```python
from build123d import *

# Parameters (mm, degrees)
CROQUIS1_R              = 2.2
SALIENTE_EXTRUIR1_DEPTH = 8.3
CORTAR_EXTRUIR1_DEPTH   = 10
CROQUIS3_R              = 11.19
CROQUIS3_R_2            = 2.2
SALIENTE_EXTRUIR2_DEPTH = 3
REDONDEO1_R             = 10
REDONDEO2_R             = 10


with BuildPart() as part:
    # Croquis1 → Saliente-Extruir1 (new body)
    with BuildSketch(Plane.XY):
        with BuildLine():
            ThreePointArc((-1.855132773, 21.210566025), (0.747663665, 19.413438157), (3.480969897, 21.005058374))
            ThreePointArc((3.480969897, 21.005058374), (4.187425829, 21.678765959), (5.158862158, 21.775064198))
            ThreePointArc((5.158862158, 21.775064198), (8.457254598, 20.718159287), (11.553044037, 19.164927682))
            ThreePointArc((11.553044037, 19.164927682), (12.17958806, 18.416325998), (12.212774884, 17.4406926))
            ThreePointArc((12.212774884, 17.4406926), (13.051461105, 14.390967482), (16.16836891, 13.853283925))
            ThreePointArc((16.16836891, 13.853283925), (17.142596439, 13.915272757), (17.948659156, 13.364614252))
            ThreePointArc((17.948659156, 13.364614252), (19.796008974, 10.434812326), (21.16912324, 7.255032793))
            ThreePointArc((21.16912324, 7.255032793), (21.16789192, 6.278835898), (20.566189442, 5.510125275))
            ThreePointArc((20.566189442, 5.510125275), (19.248334843, 2.634803184), (21.290408418, 0.219403966))
            ThreePointArc((21.290408418, 0.219403966), (22.076555656, -0.359331218), (22.340079057, -1.299287234))
            ThreePointArc((22.340079057, -1.299287234), (21.871990743, -4.731099292), (20.879934411, -8.049572571))
            ThreePointArc((20.879934411, -8.049572571), (20.251503896, -8.796591301), (19.296455393, -8.998690904))
            ThreePointArc((19.296455393, -8.998690904), (16.438698786, -10.354214806), (16.450429211, -13.517137548))
            ThreePointArc((16.450429211, -13.517137548), (16.680649129, -14.465800124), (16.278327685, -15.355237783))
            ThreePointArc((16.278327685, -15.355237783), (13.713824964, -17.683276971), (10.820792216, -19.587693468))
            ThreePointArc((10.820792216, -19.587693468), (9.859212129, -19.755995666), (8.997695409, -19.2969196))
            ThreePointArc((8.997695409, -19.2969196), (5.937212872, -18.498380614), (3.91311135, -20.928860176))
            ThreePointArc((3.91311135, -20.928860176), (3.479681489, -21.803560382), (2.599765876, -22.226301918))
            ThreePointArc((2.599765876, -22.226301918), (-0.861191929, -22.361252828), (-4.301518916, -21.960514898))
            ThreePointArc((-4.301518916, -21.960514898), (-5.146314566, -21.471350096), (-5.511186255, -20.565905154))
            ThreePointArc((-5.511186255, -20.565905154), (-7.34236093, -17.986948546), (-10.455194801, -18.54773653))
            ThreePointArc((-10.455194801, -18.54773653), (-11.349467792, -18.939192417), (-12.29525528, -18.697432369))
            ThreePointArc((-12.29525528, -18.697432369), (-15.033247546, -16.576149969), (-17.411101542, -14.057767343))
            ThreePointArc((-17.411101542, -14.057767343), (-17.743823481, -13.140021189), (-17.44132262, -12.211875121))
            ThreePointArc((-17.44132262, -12.211875121), (-17.186362452, -9.059223351), (-19.931399108, -7.487920827))
            ThreePointArc((-19.931399108, -7.487920827), (-20.868074958, -7.212965835), (-21.437189843, -6.419826415))
            ThreePointArc((-21.437189843, -6.419826415), (-22.171079561, -3.034882316), (-22.373836253, 0.422765786))
            ThreePointArc((-22.373836253, 0.422765786), (-22.038800189, 1.339669668), (-21.210470293, 1.856227))
            ThreePointArc((-21.210470293, 1.856227), (-18.988673977, 4.107413132), (-20.08148026, 7.075576251))
            ThreePointArc((-20.08148026, 7.075576251), (-20.622277928, 7.888287624), (-20.548425031, 8.861687667))
            ThreePointArc((-20.548425031, 8.861687667), (-18.934817045, 11.926440502), (-16.867604324, 14.705482106))
            ThreePointArc((-16.867604324, 14.705482106), (-16.021577354, 15.192514199), (-15.055003187, 15.055779879))
            ThreePointArc((-15.055003187, 15.055779879), (-11.905973913, 15.352145362), (-10.835213617, 18.328332564))
            ThreePointArc((-10.835213617, 18.328332564), (-10.727087865, 19.298523636), (-10.044823777, 19.996719603))
            ThreePointArc((-10.044823777, 19.996719603), (-6.838743197, 21.307249261), (-3.468832869, 22.107339915))
            ThreePointArc((-3.468832869, 22.107339915), (-2.507680415, 21.936612489), (-1.855132773, 21.210566025))
        make_face()
        with Locations(Location((0, 0, 0), (0, 0, 180))):
            Circle(CROQUIS1_R, mode=Mode.SUBTRACT)
    extrude(amount=SALIENTE_EXTRUIR1_DEPTH)

    # Croquis2 → Cortar-Extruir1 (cut)
    with BuildSketch(Plane.XY.offset(8.3)):
        Polygon((7.216878365, 0), (3.608439182, 6.25), (-3.608439182, 6.25), (-7.216878365, 0), (-3.608439182, -6.25), (3.608439182, -6.25), align=None)
    extrude(amount=-CORTAR_EXTRUIR1_DEPTH, mode=Mode.SUBTRACT)

    # Croquis3 → Saliente-Extruir2 (add)
    with BuildSketch(Plane(origin=(0, 0, 0), x_dir=(-1, 0, 0), z_dir=(0, 0, -1))):
        with Locations(Location((0, 0, 0), (0, 0, 180))):
            Circle(CROQUIS3_R)
        Circle(CROQUIS3_R_2, mode=Mode.SUBTRACT)
    extrude(amount=SALIENTE_EXTRUIR2_DEPTH)

    # Redondeo1
    # the kernel refuses this fillet: 10 mm, written as the material it adds along each edge
    with BuildSketch(Plane(origin=(0, 0, 0), x_dir=(1, 0, 0), z_dir=(0, 1, 0))) as redondeo1_piece_1:
        with BuildLine():
            CenterArc((18.331428429, 10), REDONDEO1_R, 224.427004001, 45.572995999)
            Line((11.19, 3), (11.047171431, 2.86))
            ThreePointArc((11.047171431, 2.86), (10.99, 1.5), (10.99, 0))
            Line((10.99, 0), (11.19, -0.2))
            Line((11.19, -0.2), (18.331428429, -0.2))
            Line((18.331428429, -0.2), (18.331428429, 0))
        make_face()
    revolve(axis=Axis((0, 0, 0), (0, 0, -1)))

    # Redondeo2
    redondeo2_edges = [part.edges().sort_by_distance(p)[0] for p in [
        (-11.19, 0, -3),
    ]]
    fillet(redondeo2_edges, radius=REDONDEO2_R)


solid = part.part
```
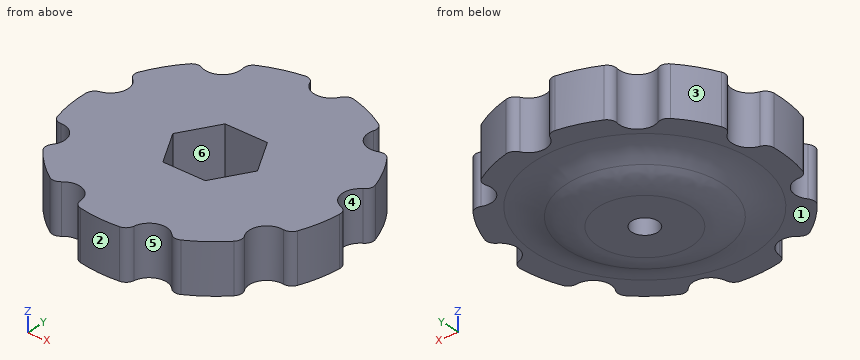
Part model, mm, in its own coordinate system. Face numbers are marked on the shaded views. A direction names the side the tool comes from. Give positions to 0.01 mm unless a question says otherwise; leave off trailing zeros. Put each result on its own line as item: value. Start each with the question number.
Item 1: Pin check, flat tips, straight feed: pin 1 Ø12 at (x, y) = (-10.5, 2) entering from -Z; pin 2 Ø2 at (x, z) = (-1, 5.5) entering from +Y; pin 3 Ø2 at (y, z) = (11, 6.5) entering from -X; pin 4 Ø4 at (x, y) = (0.5, 0) entering from +Z. Stop position of each tip, or through.
Item 2: Wall check: L1, parallel to Y at x = 0, z = -2.25; L2, parallel to X at y = -5, z = 5.25; L3, parallel to Z at x = -10.5, y = -18.5. Give the ranges that are in metal, low to high. Write a range as [from, to].
Item 3: Which spindle directions (+Z, -Z, +X, -X, +Y, -Y) get a long thin tool onto all of the face, cutting with end or side? Do the marked faces 5 and 6. Say none if no direction does.
Item 4: Pull direction Y, two halves, no side cores. Call the marked faces 1, 2, 3 and 4: pulls with the +Y half, pulls with the -Y half, needs draft (parallel to the pull), parting line crosses it, or undercut.
Answer list:
1. pin 1: stops at z = -3
1. pin 2: stops at y = 21.47
1. pin 3: stops at x = -20.02
1. pin 4: stops at z = 0
2. L1: y = [-11.6, -2.2], [2.2, 11.6]
2. L2: x = [-21.81, -4.33], [4.33, 21.81]
2. L3: z = [0, 8.3]
3. face 5: +Z, -Z, -Y
3. face 6: +Z
4. face 1: needs draft
4. face 2: pulls with the -Y half
4. face 3: pulls with the +Y half
4. face 4: undercut
